For this review, take the finished solid that the model builds, in its own axes (mm). A direction names the side the tool comes from. Coordinates: 2 decimals unless noted, no trailing zeros. Write each loop counter-clockwise with the first axis right and the second up, starting at its lowest first coordinate (ties: lowest second). Pieces come first, ordered by that corner, then holes. Notation, with made-up numbers: (-12.5, 87) - (2.5, 87) arc R18 ccw to (2.5, 102) - close; hole circle Ø6 at (28, 64.25). An arc over 180 degrees is marked (long way). Use one line per item in the form item = value. Start each with the question number.
1) Mouldability with a two-part tool opening along Z and no side actions: class faces 3 (the flat face through (31, 17, -50.381)), 4 (the flat face through (-28, 50.8, -45)), 5 (the flat face through (4, 0, 1)), 6 (the cylindrical face through (-24.378, 25.756, 42.338)) as pulls with the +Z half, pulls with the -Z half, needs draft (parallel to the pull), parting line crosses it, or undercut.
2) We need section D-D (x = -15). Give the boundary of the cut face in (y, z), plus the area to 3 significant figures.
3) We need section B-B (x = 32.5). Give the boundary of the cut face in (y, z), plus the area to 3 significant figures.
4) We need section A-A (y = 38). Count the separate pieces of the cut face and the enclosed holes in it, plus the area to 3 significant figures.
5) Tool access review of faces 1 (the flat face through (-28, 50.8, 46)), 2 (the cylindrical face through (-24.38, 25.76, -41.5)): name each direction out of +Z, -Z, +X, -X, +Y, -Y from which nothing blocks a thin tool from reaching the whole face with its end or side.
6) Insertion check: P1, Ø1.5, axis at x = 23, z = -33, coming from the +Y side. The pin has a flat end and moves straight along its axis. Give the tip position at first contact, or say it passes through.
7) We need section C-C (z = 44). Give the boundary of the cut face in (x, y), plus the area to 3 significant figures.
8) For L1, parallel to Y at x = 25, z = 35.5; L2, parallel to Z at x = -25.5, y = 38; L3, parallel to Z at x = -30, y = 4, list the stretches that pass through material, from the lowest coordinate up. Write a range as from..to.
```python
from build123d import *

# Parameters (mm, degrees)
F0_W     = 76.2
F0_H     = 101.6
F1_DEPTH = 3.81
F2_W     = 12.7
F2_H     = 12.7
F3_DEPTH = 50.8
F4_R     = 12.69999


# Not quite as in the source:
# - a fillet or chamfer is up to 0.001 mm smaller than in the source, because OpenCascade refuses the exact size


with BuildPart() as f1:
    # F0 (on Front) → F1 (new body)
    with BuildSketch(Plane.XZ):
        with Locations((4.643493332, 0.4188035619)):
            Rectangle(F0_W, F0_H)
    extrude(amount=F1_DEPTH)

    # F2 (on face) → F3 (join)
    with BuildSketch(Plane(origin=(0, 0, 0), x_dir=(-1, 0, 0), z_dir=(0, 1, 0))):
        with Locations((27.106506668, -44.0311964381)):
            Rectangle(F2_W, F2_H)
        with Locations((-36.393493332, 44.8688035619)):
            Rectangle(F2_W, F2_H)
        with Locations((27.106506668, 44.8688035619)):
            Rectangle(F2_W, F2_H)
        with Locations((-36.393493332, -44.0311964381)):
            Rectangle(F2_W, F2_H)
    extrude(amount=F3_DEPTH)

    # F4 (radius 12.7 in the source; OpenCascade refuses exactly that, so slightly less here)
    f4_edges = [f1.edges().sort_by_distance(p)[0] for p in [
        (-20.756507, 25.4, 38.518804),
        (-20.756507, 25.4, -37.681196),
        (30.043493, 25.4, -37.681196),
        (30.043493, 25.4, 38.518804),
    ]]
    fillet(f4_edges, radius=F4_R)


solid = f1.part
```
Determined:
q1.face_3 = pulls with the -Z half
q1.face_4 = needs draft
q1.face_5 = undercut
q1.face_6 = undercut
q2.outline = (-3.81, -50.38) - (0, -50.38) - (0, 51.22) - (-3.81, 51.22) - close
q2.area = 387 mm²
q3.outline = (-3.81, -50.38) - (50.8, -50.38) - (50.8, -42.87) - (0, -42.87) - (0, 43.71) - (50.8, 43.71) - (50.8, 51.22) - (-3.81, 51.22) - close
q3.area = 1,150 mm²
q4.separate_pieces = 4
q4.enclosed_holes = 0
q4.area = 507 mm²
q5.face_1 = +Z, -Z, +X, -X, +Y
q5.face_2 = +Y
q6.P1 = 0
q7.outline = (-33.46, -3.81) - (42.74, -3.81) - (42.74, 50.8) - (32.29, 50.8) - (32.29, 0) - (-23.01, 0) - (-23.01, 50.8) - (-33.46, 50.8) - close
q7.area = 1,350 mm²
q8.L1 = -3.81..0
q8.L2 = -50.38..-40.48, 41.32..51.22
q8.L3 = -50.38..-38.16, 39..51.22
